Work out the finished part from the listing and answer in its coordinate system (mm). A direction names the side the tool comes from. Coordinates: 2 decimals unless noted, no trailing zeros. Write each loop counter-clockwise with the first axis right and the second up, starting at its lowest first coordinate (ties: lowest second). Pieces come first, ordered by that corner, then holes. Notation, with made-up numbers: M 24,48.5 L 36,48.5 A33 cw 36,81.5 Z; hole C 89.5,80 d6. An arc over 180 degrees is marked long. Answer as CSV lines item,"result". Start each with the question number.
(1) The mould has two halves that part along Z. Classify faces 1 (the flat face through (39, 0, 16)), 2 (the cylindrical face through (34.6, 14.5, 6.5)), 3 (the flat face through (37, 12.297, 13)): released by +Z, released by -Z, zero draft, split by the parting line, or undercut.
(2) A cutting plane is placed at B-B on y = -9. Give the vertices of the cut face in (x, z).
(3) Find the intervals of material crossed by L1, parallel to Y at x = 26, z = 11.5; L2, parallel to Y at x = 17, z = 14; L3, parallel to X at y = -12, z = 12.5, in increasing order. Write a range as [from, to].
(4) A flat-ended cylindrical pin translates along its axis: P1, Ø1.8, axis at x = 27, y = 15.5, coming from the +Z side. Find the tip coordinate at first contact, or state that the pin passes through.
(5) A cutting plane is placed at A-A on x = 23. Give the vertices of the cut face in (y, z), then the cut area to 3 significant figures.
(6) A cutting plane is placed at C-C on z = 14.25. Count the separate pieces of the cut face and the enclosed holes in it, then the cut area to 3 significant figures.
(7) A cutting plane is placed at D-D on x = 40. Give the vertices of the cut face in (y, z).
(8) For faces 4 (the cylindrical face through (-30.283, -14.084, 10.084)), 5 (the cylindrical face through (-36.9, 16.93, 8.11)), 6 (the flat face through (32.997, 15, 14)), 7 (the flat face through (-31.5, 15, 12)), determine the directions among +Z, -Z, +X, -X, +Y, -Y from which every point of the face is accessible in a straight line to the end or side of a thin tool.
from build123d import *

# Parameters (mm, degrees)
SKETCH1_W           = 75
SKETCH1_H           = 35
BOSS_EXTRUDE5_DEPTH = 16
CUT_EXTRUDE1_DEPTH  = 12.5
CUT_EXTRUDE2_REACH  = 56.886
CUT_EXTRUDE3_DEPTH  = 7
SKETCH6_W           = 16
SKETCH6_H           = 35
BOSS_EXTRUDE6_DEPTH = 5
CUT_EXTRUDE4_DEPTH  = 58.334544561
SKETCH8_R           = 1.5
CUT_EXTRUDE5_DEPTH  = 13
SKETCH10_W          = 3
SKETCH10_H          = 5.75
CUT_EXTRUDE6_DEPTH  = 9
FILLET1_R           = 2
SKETCH11_R          = 1.8
CUT_EXTRUDE7_DEPTH  = 12


with BuildPart() as part:
    # Sketch1 → Boss-Extrude5 (new body)
    with BuildSketch(Plane.XY):
        Rectangle(SKETCH1_W, SKETCH1_H)
    extrude(amount=BOSS_EXTRUDE5_DEPTH)

    # Sketch2 → Cut-Extrude1 (cut)
    with BuildSketch(Plane.XY.offset(16)):
        Polygon((-35.5, 11.75), (-16.5, 11.75), (-16.5, 16.75), (-13.5, 16.75), (-13.5, 11.75), (-12, 11.75), (-12, -11.75), (-13.5, -11.75), (-13.5, -16.75), (-16.5, -16.75), (-16.5, -11.75), (-35.5, -11.75), align=None)
    extrude(amount=-CUT_EXTRUDE1_DEPTH, mode=Mode.SUBTRACT)

    # Sketch3 → Cut-Extrude2 (cut, up to next)
    with BuildSketch(Plane.ZY.offset(12), mode=Mode.PRIVATE) as cut_extrude2_sk1:
        with BuildLine():
            Line((9.5, 12.296655642), (16, 12.296655642))
            Line((16, 12.296655642), (16, -1.703344358))
            Line((16, -1.703344358), (9.5, -1.703344358))
            ThreePointArc((9.5, -1.703344358), (2.5, 5.296655642), (9.5, 12.296655642))
        make_face()
    cut_extrude2_tool1 = extrude(cut_extrude2_sk1.sketch, amount=-CUT_EXTRUDE2_REACH, mode=Mode.PRIVATE) & part.part
    add(cut_extrude2_tool1.solids().sort_by_distance((-12, 5.296656, 9.899379))[0], mode=Mode.SUBTRACT)

    # Sketch5 → Cut-Extrude3 (cut)
    with BuildSketch(Plane.ZY.offset(12)):
        with BuildLine():
            Line((9.702025117, -4.799998018), (16, -4.799998018))
            Line((16, -4.799998018), (16, 3.200001982))
            Line((16, 3.200001982), (9.702025117, 3.200001982))
            ThreePointArc((9.702025117, 3.200001982), (5.702025117, -0.799998018), (9.702025117, -4.799998018))
        make_face()
    extrude(amount=-CUT_EXTRUDE3_DEPTH, mode=Mode.SUBTRACT)

    # Sketch6 → Boss-Extrude6 (add)
    with BuildSketch(Plane(origin=(37.5, 0, 0), x_dir=(0, 0, -1), z_dir=(1, 0, 0))):
        with Locations((-8, 0)):
            Rectangle(SKETCH6_W, SKETCH6_H)
    extrude(amount=BOSS_EXTRUDE6_DEPTH)

    # Sketch7 → Cut-Extrude4 (cut, through all)
    with BuildSketch(Plane.XZ.offset(17.5)):
        with BuildLine():
            Line((32.99668066, 12.098076211), (32.99668066, 16))
            Line((32.99668066, 16), (35.99668066, 16))
            Line((35.99668066, 16), (35.99668066, 12.098076211))
            ThreePointArc((35.99668066, 12.098076211), (34.49668066, 6.5), (32.99668066, 12.098076211))
        make_face()
    extrude(amount=-CUT_EXTRUDE4_DEPTH, mode=Mode.SUBTRACT)

    # Sketch8 → Cut-Extrude5 (cut)
    with BuildSketch(Plane.XY.offset(16)):
        with Locations((40, 15)):
            Circle(SKETCH8_R)
    extrude(amount=-CUT_EXTRUDE5_DEPTH, mode=Mode.SUBTRACT)

    # Sketch10 → Cut-Extrude6 (cut)
    with BuildSketch(Plane.XY.offset(16)):
        with Locations((-30, 14.625)):
            Rectangle(SKETCH10_W, SKETCH10_H)
    extrude(amount=-CUT_EXTRUDE6_DEPTH, mode=Mode.SUBTRACT)

    # Fillet1
    fillet1_edges = [part.edges().sort_by_distance(p)[0] for p in [
        (-37.5, -17.5, 8),
        (-37.5, 17.5, 8),
    ]]
    fillet(fillet1_edges, radius=FILLET1_R)

    # Sketch11 → Cut-Extrude7 (cut)
    with BuildSketch(Plane.XY.offset(16)):
        with Locations((-32, -14.625)):
            Circle(SKETCH11_R)
        with Locations((26, 14.898327821)):
            Circle(SKETCH11_R)
    extrude(amount=-CUT_EXTRUDE7_DEPTH, mode=Mode.SUBTRACT)


solid = part.part
Here are the results:
1,face 1,"released by +Z"
1,face 2,"undercut"
1,face 3,"zero draft"
2,outline,"M -37.5,0 L 42.5,0 L 42.5,16 L 36,16 L 36,12.1 A3 cw long 33,12.1 L 33,16 L -12,16 L -12,3.5 L -35.5,3.5 L -35.5,16 L -37.5,16 Z"
3,L1,"y = [-17.5, -1.7], [12.3, 13.1], [16.7, 17.5]"
3,L2,"y = [-17.5, -1.7], [12.3, 17.5]"
3,L3,"x = [-37.5, -16.5], [-13.5, 33], [36, 42.5]"
4,P1,"stops at z = 16"
5,outline,"M -17.5,0 L 17.5,0 L 17.5,16 L 12.3,16 L 12.3,9.5 A7 cw -1.7,9.5 L -1.7,16 L -17.5,16 Z"
5,area,"392 mm^2"
6,separate pieces,"3"
6,enclosed holes,"3"
6,area,"1,390 mm^2"
7,outline,"M -17.5,0 L 17.5,0 L 17.5,16 L 16.5,16 L 16.5,3 L 13.5,3 L 13.5,16 L -17.5,16 Z"
8,face 4,"+Z"
8,face 5,"+Z, -Z, -X, +Y"
8,face 6,"+Z, +Y, -Y"
8,face 7,"+Z, +Y"
